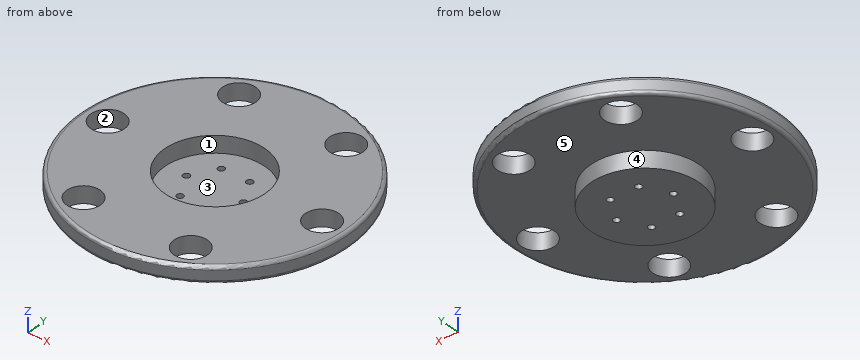
from build123d import *

# Parameters (mm, degrees)
SKETCH_2_R          = 80
EXTRUDE_1_DEPTH     = 10
SKETCH_3_R          = 32.5
EXTRUDE_2_DEPTH     = 10
SKETCH_4_R          = 2
CUT_EXTRUDE_1_DEPTH = 10
SKETCH_5_R          = 30
CUT_EXTRUDE_2_DEPTH = 10
SKETCH_6_R          = 10
CUT_EXTRUDE_3_DEPTH = 10
FILLET_1_R          = 2


with BuildPart() as part:
    # 草图2 → 凸台-拉伸1 (new body)
    with BuildSketch(Plane.XY):
        Circle(SKETCH_2_R)
    extrude(amount=EXTRUDE_1_DEPTH)

    # 草图3 → 凸台-拉伸2 (add)
    with BuildSketch(Plane.XY):
        Circle(SKETCH_3_R)
    extrude(amount=-EXTRUDE_2_DEPTH)

    # 草图4 → 切除-拉伸1 (cut)
    with BuildSketch(Plane.XY):
        with Locations((-17.25, 0)):
            Circle(SKETCH_4_R)
        with Locations((-8.625, 14.938938215)):
            Circle(SKETCH_4_R)
        with Locations((8.625, 14.938938215)):
            Circle(SKETCH_4_R)
        with Locations((17.25, 0)):
            Circle(SKETCH_4_R)
        with Locations((8.625, -14.938938215)):
            Circle(SKETCH_4_R)
        with Locations((-8.625, -14.938938215)):
            Circle(SKETCH_4_R)
    extrude(amount=-CUT_EXTRUDE_1_DEPTH, mode=Mode.SUBTRACT)

    # 草图5 → 切除-拉伸2 (cut)
    with BuildSketch(Plane.XY):
        Circle(SKETCH_5_R)
    extrude(amount=CUT_EXTRUDE_2_DEPTH, mode=Mode.SUBTRACT)

    # 草图6 → 切除-拉伸3 (cut)
    with BuildSketch(Plane.XY):
        with Locations((-65, 0)):
            Circle(SKETCH_6_R)
        with Locations((-32.5, 56.291651246)):
            Circle(SKETCH_6_R)
        with Locations((32.5, 56.291651246)):
            Circle(SKETCH_6_R)
        with Locations((65, 0)):
            Circle(SKETCH_6_R)
        with Locations((32.5, -56.291651246)):
            Circle(SKETCH_6_R)
        with Locations((-32.5, -56.291651246)):
            Circle(SKETCH_6_R)
    extrude(amount=CUT_EXTRUDE_3_DEPTH, mode=Mode.SUBTRACT)

    # 圆角1
    fillet_1_edges = [part.edges().sort_by_distance(p)[0] for p in [
        (-80, 0, 0),
        (-80, 0, 10),
    ]]
    fillet(fillet_1_edges, radius=FILLET_1_R)


solid = part.part
Verification items for the finished model (mm, model axes). Face numbers are marked on the shaded views. A direction names the side the tool comes from. Round coordinates to 2 decimals unless told otherwise and drop trailing zeros. Order: outer loops, then holes, each group sorted by start corner. A loop starts at its lowest first (then second) coordinate and runs counter-clockwise, first axis right, second up.
1. Section check B-B on x = 0. Record the cut outline in (y, z).
Final values:
outline: (-80, 2) arc R2 ccw to (-78, 0) - (-32.5, 0) - (-32.5, -10) - (32.5, -10) - (32.5, 0) - (78, 0) arc R2 ccw to (80, 2) - (80, 8) arc R2 ccw to (78, 10) - (30, 10) - (30, 0) - (-30, 0) - (-30, 10) - (-78, 10) arc R2 ccw to (-80, 8) - close
2. Go/stop test with flat-tipped pins: P1, Ø6.5, axis at x = -8.62, y = 14.94, coming from the +Z side; P2, Ø5, axis at x = 34, z = 1.5, coming from the +Y side; P3, Ø5, axis at x = -28.5, z = 3.5, coming from the +Y side. Record where each tip stops, or that it passes through.
Final values:
P1: stops at z = 0
P2: stops at y = 73.52
P3: stops at y = 75.66
3. Release check for a two-part mould opening along Y. For the marked faces 3, 4 and 5 record: +Y half, -Y half, draft (parallel to the pull), parting line (faces both ways), or undercut.
Final values:
face 3: undercut
face 4: parting line
face 5: draft
4. Access from +Z, -Z, +X, -X, +Y, -Y to the whole of each face (thin tool, end or side, straight path). Record for the marked faces 1 and 2.
Final values:
face 1: +Z
face 2: +Z, -Z
5. Thickness scan on L1, parallel to Y at x = 0, z = 4.25; L2, parallel to X at y = 13, z = 2; L3, parallel to X at y = 57, z = 5. Record the ranges inside material, lowest first.
Final values:
L1: y = -80 to -30, 30 to 80
L2: x = -78.94 to -27.04, 27.04 to 78.94
L3: x = -56.13 to -42.47, -22.53 to 22.53, 42.47 to 56.13
6. Section check C-C on z = -3. Record the cut outline in (x, y) (3 decimals).
Final values:
outline: circle Ø65 at (0, 0); hole circle Ø4 at (-17.25, 0); hole circle Ø4 at (-8.625, -14.939); hole circle Ø4 at (-8.625, 14.939); hole circle Ø4 at (8.625, -14.939); hole circle Ø4 at (8.625, 14.939); hole circle Ø4 at (17.25, 0)
7. Section check A-A on y = 0. State how many separate pieces and enclosed holes the cut face has, then the cut area to 3 significant figures.
Final values:
separate pieces: 5
enclosed holes: 0
area: 1,170 mm2
